Verification items for the finished model (mm, model axes). A direction names the side the tool comes from. Give positions to 0.01 mm unless a question says otherwise; leave off trailing zeros. Order: outer loops, then holes, each group sorted by start corner. A loop starts at its lowest first (then second) coordinate and runs counter-clockwise, first axis right, second up. Notation, with made-up numbers: (-4, 69) -> (1, 69) arc R23 cw to (1, 81) -> close; hole circle Ø10 at (-26, 69.25). An arc over 180 degrees is marked (long way). One line per question, with ' | ' between items. Start each with the question number.
Q1. Section check D-D on y = -11. Record the cut outline in (x, z), plus the area to 3 significant figures.
Q2. Go/stop test with flat-tipped pins: pin 1 (5 mm diameter, centred on x = 14, y = -27.5, fed in from -Z); pin 2 (1.5 mm diameter, centred on y = -7.5, z = 1, fed in from +X); pin 3 (1.6 mm diameter, centred on x = 10, y = -48.5, fed in from +Z); pin 4 (1.6 mm diameter, centred on x = 10.5, y = -4.5, fed in from +Z). Record where each tip stops, or that it passes through.
Q3. Section check C-C on x = 10. Give the number of separate pieces and of enclosed holes in the cut face, plus the area to 3 significant figures.
Q4. Access from +Z, -Z, +X, -X, +Y, -Y to the whole of each face (thin tool, end or side, straight path). Record for faces 4 (the cylindrical face through (6.71, -13.53, 2.37)), 5 (the flat face through (12, -48, 1.8)).
Q5. Section check B-B on z = 4.3. Record the cut outline in (x, y), plus the area to 3 significant figures.
Q6. Mould release check, pull along Y, two halves, no side actions. Record for faces 1 (the flat face through (6, -26, 0)), 2 (the flat face through (13, -52, 2)), 3 (the cylindrical face through (11.246, -50.895, 3.279)): released by +Y, released by -Y, zero draft, split by the parting line, or undercut.
Q7. Section check A-A on y = -3.5. Record the cut outline in (x, z).
Q8. Material ranges on probe 1 along Y at (x, z) = (10, 2.35); probe 2 along Y at (x, z) = (10, 1.3); probe 3 along X at (y, z) = (-26, 0.3), recorded low to high. Write a range as [from, to].
from build123d import *

# Parameters (mm, degrees)
CYLINDER1006_R     = 4.15
CYLINDER1006_DEPTH = 70
CYLINDER1020_R     = 2.7
CYLINDER1020_DEPTH = 10
CYLINDER1018_R     = 1.7
CYLINDER1018_DEPTH = 10
CYLINDER1032_R     = 3.5
CYLINDER1032_DEPTH = 10
PAD021_DEPTH       = 52


with BuildPart() as obj1:
    # Cylinder1006 → Cylinder1006 (new body)
    with BuildSketch(Plane.XY):
        Circle(CYLINDER1006_R)
    extrude(amount=CYLINDER1006_DEPTH)


with BuildPart() as obj2:
    # Clone046 base: copy of obj1
    add(obj1.part)


with BuildPart() as obj2_1:
    # Clone046 placement: moved
    add(obj2.part.moved(Location((10, -11, -55.2))))


with BuildPart() as cylinder1015:
    # Cylinder1020 → Cylinder1020 (new body)
    with BuildSketch(Plane.XY.offset(10)):
        Circle(CYLINDER1020_R)
    extrude(amount=CYLINDER1020_DEPTH)


with BuildPart() as m3bolthead:
    # Cylinder1018 → Cylinder1018 (new body)
    with BuildSketch(Plane.XY):
        Circle(CYLINDER1018_R)
    extrude(amount=CYLINDER1018_DEPTH)

    # Fusion024: union Cylinder1015
    add(cylinder1015.part)


with BuildPart() as clone_of_m3bolthead005:
    # Clone047 base: copy of M3BoltHead
    add(m3bolthead.part)


with BuildPart() as clone_of_m3bolthead005_1:
    # Clone047 placement: moved
    add(clone_of_m3bolthead005.part.moved(Location((10, -3.5, -8.2))))


with BuildPart() as clone_of_m3bolthead006:
    # Clone048 base: copy of M3BoltHead
    add(m3bolthead.part)


with BuildPart() as clone_of_m3bolthead006_1:
    # Clone048 placement: moved
    add(clone_of_m3bolthead006.part.moved(Location((10, -48.5, -8.2))))


with BuildPart() as cylinder1046:
    # Cylinder1032 → Cylinder1032 (new body)
    with BuildSketch(Plane(origin=(10, -26, -4.4), x_dir=(1, 0, 0), z_dir=(0, 0, 1))):
        Circle(CYLINDER1032_R)
    extrude(amount=CYLINDER1032_DEPTH)


with BuildPart() as fusion049:
    # Clone045 base: copy of obj1
    add(obj1.part)


with BuildPart() as fusion049_1:
    # Clone045 placement: moved
    add(fusion049.part.moved(Location((10, -41, -55.2))))

    # Fusion049: union obj2, Clone of M3BoltHead005, Clone of M3BoltHead006, Cylinder1046
    add(obj2_1.part)
    add(clone_of_m3bolthead005_1.part)
    add(clone_of_m3bolthead006_1.part)
    add(cylinder1046.part)


with BuildPart() as obj3:
    # Sketch022 → Pad021 (new body)
    with BuildSketch(Plane.XZ):
        Polygon((0, 0), (0, 4.8), (24.8, 4.8), (20, 0), align=None)
    extrude(amount=PAD021_DEPTH)

    # Cut051: cut Fusion049
    add(fusion049_1.part, mode=Mode.SUBTRACT)


solid = obj3.part
Filled in:
1) outline: (0, 0) -> (5.85, 0) -> (5.85, 4.8) -> (0, 4.8) -> close; (14.15, 0) -> (20, 0) -> (24.8, 4.8) -> (14.15, 4.8) -> close | area: 67.7 mm²
2) pin 1: z = 0 | pin 2: x = 21.75 | pin 3: through | pin 4: z = 1.8
3) separate pieces: 6 | enclosed holes: 0 | area: 91.7 mm²
4) face 4: +Z, -Z | face 5: +Z
5) outline: (0, -52) -> (24.3, -52) -> (24.3, 0) -> (0, 0) -> close; hole circle Ø8.3 at (10, -41); hole circle Ø8.3 at (10, -11); hole circle Ø7 at (10, -26); hole circle Ø5.4 at (10, -48.5); hole circle Ø5.4 at (10, -3.5) | area: 1,070 mm²
6) face 1: zero draft | face 2: released by -Y | face 3: undercut
7) outline: (0, 0) -> (8.3, 0) -> (8.3, 1.8) -> (7.3, 1.8) -> (7.3, 4.8) -> (0, 4.8) -> close; (11.7, 0) -> (20, 0) -> (24.8, 4.8) -> (12.7, 4.8) -> (12.7, 1.8) -> (11.7, 1.8) -> close
8) probe 1: [-52, -51.2], [-45.8, -45.15], [-36.85, -29.5], [-22.5, -15.15], [-6.85, -6.2], [-0.8, 0] | probe 2: [-52, -50.2], [-46.8, -45.15], [-36.85, -29.5], [-22.5, -15.15], [-6.85, -5.2], [-1.8, 0] | probe 3: [0, 6.5], [13.5, 20.3]
